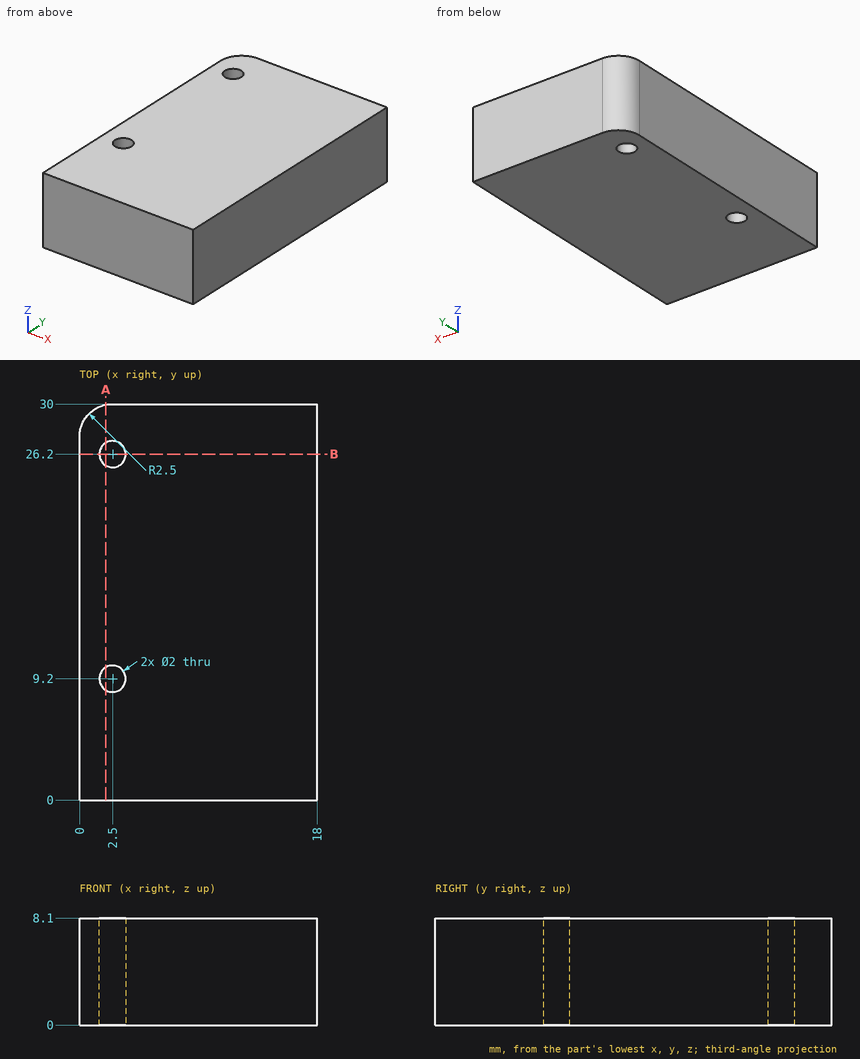
Part print with two shaded views. Sizes in mm from the minimum x, y, z corner. Give positions to 0.01 mm unless a question says otherwise; leave off trailing zeros. Order: outer loops, then holes, each group sorted by start corner. A loop starts at its lowest first (then second) coordinate and runs counter-clockwise, first axis right, second up.
(1) Saw through at A-A, the plane x = 2. Give the cut face in (y, z), then the cut area to 3 significant figures.
(2) Saw through at B-B, the plane y = 26.2. Give the cut face in (x, z).
(3) Flat gauge pin, fed straight in: pin 1 (3 mm diameter, centred on x = 2.5, y = 26.2, fed in from -Z). Where does the tip first touch, or does it go through?
(4) Drill centre lines: L1, parallel to Y at x = 2.5, z = 3.25; L2, parallel to X at y = 8.5, z = 6; L3, parallel to X at y = 29.25, z = 1.5. Where is each one in solid material? Low to high.
Results found:
1. outline: (0, 0) - (8.33, 0) - (8.33, 8.1) - (0, 8.1) - close; (10.07, 0) - (25.33, 0) - (25.33, 8.1) - (10.07, 8.1) - close; (27.07, 0) - (29.95, 0) - (29.95, 8.1) - (27.07, 8.1) - close
1. area: 215 mm2
2. outline: (0, 0) - (1.5, 0) - (1.5, 8.1) - (0, 8.1) - close; (3.5, 0) - (18, 0) - (18, 8.1) - (3.5, 8.1) - close
3. pin 1: stops at z = 0
4. L1: y = 0 to 8.2, 10.2 to 25.2, 27.2 to 30
4. L2: x = 0 to 1.79, 3.21 to 18
4. L3: x = 0.71 to 18
